Input: part model. Units: mm. Frame: model coordinates. A direction names the side the tool comes from. Give positions to 0.01 mm unless a question says otherwise; leave off trailing zeros. Order: outer loops, then holes, each group sorted by start corner. A loop starts at its lowest first (then second) coordinate and runs counter-clockwise, first axis right, second up. Notation, with made-up numbers: M 25,-37.75 L 45,-37.75 A24 cw 45,-5.75 Z; hole C 26.5,36 d10. An arc over 180 degrees is marked long. Use a Markdown table: item, result.
from build123d import *

# Parameters (mm, degrees)
ESQUISSE1_R             = 2.5
BOSS_EXTRU_1_DEPTH      = 2
ESQUISSE2_W             = 16
ESQUISSE2_H             = 2
BOSS_EXTRU_2_DEPTH      = 42
CONG_1_R                = 1
ENL_V_MAT_EXTRU_1_REACH = 63.351
ESQUISSE3_R             = 2.5
CONG_2_SIZE             = 3
CONG_2_SIZE_2           = 8
CONG_3_SIZE             = 3
CONG_3_SIZE_2           = 8


with BuildPart() as part:
    # Esquisse1 → Boss.-Extru.1 (new body)
    with BuildSketch(Plane.XY):
        Polygon((0, 0), (8, 0), (8, 42), (-8, 42), (-8, 0), align=None)
        with Locations((0, 12)):
            Circle(ESQUISSE1_R, mode=Mode.SUBTRACT)
        with Locations((0, 34)):
            Circle(ESQUISSE1_R, mode=Mode.SUBTRACT)
    extrude(amount=BOSS_EXTRU_1_DEPTH)

    # Esquisse2 → Boss.-Extru.2 (add)
    with BuildSketch(Plane.XY.offset(2)):
        with Locations((0, 1)):
            Rectangle(ESQUISSE2_W, ESQUISSE2_H)
    extrude(amount=BOSS_EXTRU_2_DEPTH)

    # Congé1
    cong_1_edges = [part.edges().sort_by_distance(p)[0] for p in [
        (0, 2, 2),
        (0, 0, 0),
    ]]
    fillet(cong_1_edges, radius=CONG_1_R)

    # Esquisse3 → Enlèv. mat.-Extru.1 (cut, up to next)
    with BuildSketch(Plane.XZ, mode=Mode.PRIVATE) as enl_v_mat_extru_1_sk1:
        with Locations(Location((0, 12, 0), (0, 0, 270))):
            Circle(ESQUISSE3_R)
    enl_v_mat_extru_1_tool1 = extrude(enl_v_mat_extru_1_sk1.sketch, amount=-ENL_V_MAT_EXTRU_1_REACH, mode=Mode.PRIVATE) & part.part
    # Esquisse3 → Enlèv. mat.-Extru.1 (cut, up to next)
    with BuildSketch(Plane.XZ, mode=Mode.PRIVATE) as enl_v_mat_extru_1_sk2:
        with Locations(Location((0, 34, 0), (0, 0, 270))):
            Circle(ESQUISSE3_R)
    enl_v_mat_extru_1_tool2 = extrude(enl_v_mat_extru_1_sk2.sketch, amount=-ENL_V_MAT_EXTRU_1_REACH, mode=Mode.PRIVATE) & part.part
    add(enl_v_mat_extru_1_tool1.solids().sort_by_distance((0, 0, 12))[0], mode=Mode.SUBTRACT)
    add(enl_v_mat_extru_1_tool2.solids().sort_by_distance((0, 0, 34))[0], mode=Mode.SUBTRACT)

    # Congé2
    # an asymmetric fillet: 8, 3 mm, written as the material it takes off along each edge
    with BuildSketch(Plane(origin=(8, 42, -20), x_dir=(0, -1, 0), z_dir=(0, 0, 1))) as cong_2_piece_1:
        with BuildLine():
            Bezier((CONG_2_SIZE, 0), (0, 0), (0, -CONG_2_SIZE_2), weights=[1, 0.707106781, 1])
            Line((0, -CONG_2_SIZE_2), (0, 0))
            Line((0, 0), (CONG_2_SIZE, 0))
        make_face()
    extrude(amount=42, mode=Mode.SUBTRACT)
    with BuildSketch(Plane(origin=(-8, 22, 44), x_dir=(1, 0, 0), z_dir=(0, -1, 0))) as cong_2_piece_2:
        with BuildLine():
            Bezier((CONG_2_SIZE_2, 0), (0, 0), (0, -CONG_2_SIZE), weights=[1, 0.707106781, 1])
            Line((0, -CONG_2_SIZE), (0, 0))
            Line((0, 0), (CONG_2_SIZE_2, 0))
        make_face()
    extrude(amount=42, mode=Mode.SUBTRACT)
    with BuildSketch(Plane(origin=(8, -20, 44), x_dir=(0, 0, -1), z_dir=(0, 1, 0))) as cong_2_piece_3:
        with BuildLine():
            Bezier((CONG_2_SIZE, 0), (0, 0), (0, CONG_2_SIZE_2), weights=[1, 0.707106781, 1])
            Line((0, CONG_2_SIZE_2), (0, 0))
            Line((0, 0), (CONG_2_SIZE, 0))
        make_face()
    extrude(amount=42, mode=Mode.SUBTRACT)

    # Congé3
    # an asymmetric fillet: 8, 3 mm, written as the material it takes off along each edge
    with BuildSketch(Plane(origin=(-8, 42, -20), x_dir=(0, -1, 0), z_dir=(0, 0, 1))) as cong_3_piece_1:
        with BuildLine():
            Bezier((CONG_3_SIZE, 0), (0, 0), (0, CONG_3_SIZE_2), weights=[1, 0.707106781, 1])
            Line((0, CONG_3_SIZE_2), (0, 0))
            Line((0, 0), (CONG_3_SIZE, 0))
        make_face()
    extrude(amount=42, mode=Mode.SUBTRACT)


solid = part.part
1) Cut plane A-A on y = 12. Return loops of the section in (x, z).
Response values:
| item | result |
|---|---|
| outline | M -8,0 L -2.5,0 L -2.5,2 L -8,2 Z; M 2.5,0 L 8,0 L 8,2 L 2.5,2 Z |
2) Material intervals for line 1 (Z direction, x = 4, y = 22.5); line 2 (Y direction, x = 0, z = 0.5), sorted ascending. Write a range as from..to.
Response values:
| item | result |
|---|---|
| line 1 | z = 0..2 |
| line 2 | y = 0.13..9.5, 14.5..31.5, 36.5..42 |
3) Cut plane D-D on x = 1.25. State how many separate pieces and enclosed holes the cut face has, and give its area (3 significant figures).
Response values:
| item | result |
|---|---|
| separate pieces | 5 |
| enclosed holes | 0 |
| area | 133 mm² |
4) Mould query, pull axis Z, two halves, no side actions, for faces 1 (the face through (-0.54, 9.56, 0.99)), 2 (the face through (0.1, 1, 14.5)), 3 (the face through (0.112, 0.285, 0.301)), 4 (the face through (-0.96, 0.99, 31.69)). Classes: released by +Z, released by -Z, zero draft, split by the parting line, or undercut.
Response values:
| item | result |
|---|---|
| face 1 | zero draft |
| face 2 | undercut |
| face 3 | released by -Z |
| face 4 | undercut |
5) Reachability of faces 5 (the face through (0, 0, 22)), 6 (the face through (0, 2, 23)) from +Z, -Z, +X, -X, +Y, -Y: full face, straight path, thin tool, end or side. Return the list, or none.
Response values:
| item | result |
|---|---|
| face 5 | +Z, -Z, +X, -X, -Y |
| face 6 | +Z, +X, -X, +Y |
6) Cut plane C-C on y = 18.5. Return loops of the section in (x, z), and give its area (3 significant figures).
Response values:
| item | result |
|---|---|
| outline | M -8,0 L 8,0 L 8,2 L -8,2 Z |
| area | 32.0 mm² |
7) First-contact query: pin 1 Ø6.5 at (x, z) = (0, 12) entering from -Y; pin 2 Ø3 at (x, y) = (6, 18.5) entering from +Z; pin 3 Ø5 at (x, z) = (2, 31.5) entering from +Y. Flat tips, straight axial feed; report the tip coordinate or a pass-through.
Response values:
| item | result |
|---|---|
| pin 1 | stops at y = 0 |
| pin 2 | stops at z = 2 |
| pin 3 | stops at y = 2 |
